Here's how the part is built. I have some questions about the finished solid (model axes, mm). Round coordinates to 2 decimals unless told otherwise and drop trailing zeros. Loops run counter-clockwise (first coordinate to the right, second up) from the corner with the lowest first, then second, coordinate; pieces in that order, holes last. Notation, with made-up numbers: M -19,63 L 3,63 A25 ccw 3,98 Z; hole C -39.5,50 d3. An arc over 180 degrees is marked long. Answer as CSV lines item,"result".
```python
from build123d import *

# Parameters (mm, degrees)
F0_R     = 0.875
F0_R_2   = 0.475
F1_DEPTH = 1.6
F2_DEPTH = 0.25


with BuildPart() as f1:
    # F0 (on Top) → F1 (new body)
    with BuildSketch(Plane.XY):
        Polygon((-5.712371, 40.124945), (-28.712371, 40.124945), (-28.712371, 37.474945), (-28.712371, 34.824945), (-5.712371, 34.824945), (-5.712371, 37.474945), align=None)
        with Locations((-27.27286, 36.149945)):
            Circle(F0_R, mode=Mode.SUBTRACT)
        with Locations((-24.77286, 36.149945)):
            Circle(F0_R, mode=Mode.SUBTRACT)
        with Locations((-22.27286, 36.149945)):
            Circle(F0_R, mode=Mode.SUBTRACT)
        with Locations((-19.77286, 36.149945)):
            Circle(F0_R, mode=Mode.SUBTRACT)
        with Locations((-17.27286, 36.149945)):
            Circle(F0_R, mode=Mode.SUBTRACT)
        with Locations((-14.77286, 36.149945)):
            Circle(F0_R, mode=Mode.SUBTRACT)
        with Locations((-12.27286, 36.149945)):
            Circle(F0_R, mode=Mode.SUBTRACT)
        with Locations((-9.77286, 36.149945)):
            Circle(F0_R, mode=Mode.SUBTRACT)
        with Locations((-7.27286, 36.149945)):
            Circle(F0_R, mode=Mode.SUBTRACT)
        with Locations((-27.264467, 38.799945)):
            Circle(F0_R, mode=Mode.SUBTRACT)
        with Locations((-24.764467, 38.799945)):
            Circle(F0_R, mode=Mode.SUBTRACT)
        with Locations((-22.264467, 38.799945)):
            Circle(F0_R, mode=Mode.SUBTRACT)
        with Locations((-19.764467, 38.799945)):
            Circle(F0_R, mode=Mode.SUBTRACT)
        with Locations((-17.264467, 38.799945)):
            Circle(F0_R, mode=Mode.SUBTRACT)
        with Locations((-14.764467, 38.799945)):
            Circle(F0_R, mode=Mode.SUBTRACT)
        with Locations((-12.264467, 38.799945)):
            Circle(F0_R, mode=Mode.SUBTRACT)
        with Locations((-9.764467, 38.799945)):
            Circle(F0_R, mode=Mode.SUBTRACT)
        with Locations((-7.264467, 38.799945)):
            Circle(F0_R, mode=Mode.SUBTRACT)
        with Locations((-27.264467, 38.799945)):
            Circle(F0_R)
        with Locations((-27.264467, 38.799945)):
            Circle(F0_R_2, mode=Mode.SUBTRACT)
        with Locations((-24.764467, 38.799945)):
            Circle(F0_R)
        with Locations((-24.764467, 38.799945)):
            Circle(F0_R_2, mode=Mode.SUBTRACT)
        with Locations((-22.264467, 38.799945)):
            Circle(F0_R)
        with Locations((-22.264467, 38.799945)):
            Circle(F0_R_2, mode=Mode.SUBTRACT)
        with Locations((-19.764467, 38.799945)):
            Circle(F0_R)
        with Locations((-19.764467, 38.799945)):
            Circle(F0_R_2, mode=Mode.SUBTRACT)
        with Locations((-17.264467, 38.799945)):
            Circle(F0_R)
        with Locations((-17.264467, 38.799945)):
            Circle(F0_R_2, mode=Mode.SUBTRACT)
        with Locations((-14.764467, 38.799945)):
            Circle(F0_R)
        with Locations((-14.764467, 38.799945)):
            Circle(F0_R_2, mode=Mode.SUBTRACT)
        with Locations((-12.264467, 38.799945)):
            Circle(F0_R)
        with Locations((-12.264467, 38.799945)):
            Circle(F0_R_2, mode=Mode.SUBTRACT)
        with Locations((-9.764467, 38.799945)):
            Circle(F0_R)
        with Locations((-9.764467, 38.799945)):
            Circle(F0_R_2, mode=Mode.SUBTRACT)
        with Locations((-7.264467, 38.799945)):
            Circle(F0_R)
        with Locations((-7.264467, 38.799945)):
            Circle(F0_R_2, mode=Mode.SUBTRACT)
        with Locations((-7.27286, 36.149945)):
            Circle(F0_R)
        with Locations((-7.27286, 36.149945)):
            Circle(F0_R_2, mode=Mode.SUBTRACT)
        with Locations((-9.77286, 36.149945)):
            Circle(F0_R)
        with Locations((-9.77286, 36.149945)):
            Circle(F0_R_2, mode=Mode.SUBTRACT)
        with Locations((-12.27286, 36.149945)):
            Circle(F0_R)
        with Locations((-12.27286, 36.149945)):
            Circle(F0_R_2, mode=Mode.SUBTRACT)
        with Locations((-14.77286, 36.149945)):
            Circle(F0_R)
        with Locations((-14.77286, 36.149945)):
            Circle(F0_R_2, mode=Mode.SUBTRACT)
        with Locations((-17.27286, 36.149945)):
            Circle(F0_R)
        with Locations((-17.27286, 36.149945)):
            Circle(F0_R_2, mode=Mode.SUBTRACT)
        with Locations((-19.77286, 36.149945)):
            Circle(F0_R)
        with Locations((-19.77286, 36.149945)):
            Circle(F0_R_2, mode=Mode.SUBTRACT)
        with Locations((-22.27286, 36.149945)):
            Circle(F0_R)
        with Locations((-22.27286, 36.149945)):
            Circle(F0_R_2, mode=Mode.SUBTRACT)
        with Locations((-24.77286, 36.149945)):
            Circle(F0_R)
        with Locations((-24.77286, 36.149945)):
            Circle(F0_R_2, mode=Mode.SUBTRACT)
        with Locations((-27.27286, 36.149945)):
            Circle(F0_R)
        with Locations((-27.27286, 36.149945)):
            Circle(F0_R_2, mode=Mode.SUBTRACT)
    extrude(amount=-F1_DEPTH)

    # F0 (on Top) → F2 (join)
    with BuildSketch(Plane.XY):
        with Locations((-27.264467, 38.799945)):
            Circle(F0_R)
        with Locations((-27.264467, 38.799945)):
            Circle(F0_R_2, mode=Mode.SUBTRACT)
        with Locations((-24.764467, 38.799945)):
            Circle(F0_R)
        with Locations((-24.764467, 38.799945)):
            Circle(F0_R_2, mode=Mode.SUBTRACT)
        with Locations((-22.264467, 38.799945)):
            Circle(F0_R)
        with Locations((-22.264467, 38.799945)):
            Circle(F0_R_2, mode=Mode.SUBTRACT)
        with Locations((-19.764467, 38.799945)):
            Circle(F0_R)
        with Locations((-19.764467, 38.799945)):
            Circle(F0_R_2, mode=Mode.SUBTRACT)
        with Locations((-17.264467, 38.799945)):
            Circle(F0_R)
        with Locations((-17.264467, 38.799945)):
            Circle(F0_R_2, mode=Mode.SUBTRACT)
        with Locations((-14.764467, 38.799945)):
            Circle(F0_R)
        with Locations((-14.764467, 38.799945)):
            Circle(F0_R_2, mode=Mode.SUBTRACT)
        with Locations((-12.264467, 38.799945)):
            Circle(F0_R)
        with Locations((-12.264467, 38.799945)):
            Circle(F0_R_2, mode=Mode.SUBTRACT)
        with Locations((-9.764467, 38.799945)):
            Circle(F0_R)
        with Locations((-9.764467, 38.799945)):
            Circle(F0_R_2, mode=Mode.SUBTRACT)
        with Locations((-27.27286, 36.149945)):
            Circle(F0_R)
        with Locations((-27.27286, 36.149945)):
            Circle(F0_R_2, mode=Mode.SUBTRACT)
        with Locations((-24.77286, 36.149945)):
            Circle(F0_R)
        with Locations((-24.77286, 36.149945)):
            Circle(F0_R_2, mode=Mode.SUBTRACT)
        with Locations((-22.27286, 36.149945)):
            Circle(F0_R)
        with Locations((-22.27286, 36.149945)):
            Circle(F0_R_2, mode=Mode.SUBTRACT)
        with Locations((-19.77286, 36.149945)):
            Circle(F0_R)
        with Locations((-19.77286, 36.149945)):
            Circle(F0_R_2, mode=Mode.SUBTRACT)
        with Locations((-17.27286, 36.149945)):
            Circle(F0_R)
        with Locations((-17.27286, 36.149945)):
            Circle(F0_R_2, mode=Mode.SUBTRACT)
        with Locations((-14.77286, 36.149945)):
            Circle(F0_R)
        with Locations((-14.77286, 36.149945)):
            Circle(F0_R_2, mode=Mode.SUBTRACT)
        with Locations((-12.27286, 36.149945)):
            Circle(F0_R)
        with Locations((-12.27286, 36.149945)):
            Circle(F0_R_2, mode=Mode.SUBTRACT)
        with Locations((-9.77286, 36.149945)):
            Circle(F0_R)
        with Locations((-9.77286, 36.149945)):
            Circle(F0_R_2, mode=Mode.SUBTRACT)
        with Locations((-7.27286, 36.149945)):
            Circle(F0_R)
        with Locations((-7.27286, 36.149945)):
            Circle(F0_R_2, mode=Mode.SUBTRACT)
        with Locations((-7.264467, 38.799945)):
            Circle(F0_R)
        with Locations((-7.264467, 38.799945)):
            Circle(F0_R_2, mode=Mode.SUBTRACT)
    extrude(amount=F2_DEPTH)


solid = f1.part
```
1. I want a section at A-A, the plane x = -19.75. Please give me the cut outline in (y, z), and give its area (3 significant figures).
Evaluation:
outline,"M 34.82,-1.6 L 35.68,-1.6 L 35.68,0.25 L 35.28,0.25 L 35.28,0 L 34.82,0 Z; M 36.62,-1.6 L 38.33,-1.6 L 38.33,0.25 L 37.93,0.25 L 37.93,0 L 37.02,0 L 37.02,0.25 L 36.62,0.25 Z; M 39.27,-1.6 L 40.12,-1.6 L 40.12,0 L 39.67,0 L 39.67,0.25 L 39.27,0.25 Z"
area,"5.84 mm²"
2. I want a section at B-B, the plane z = -0.45. Count the separate pieces of the cut face and the enclosed holes in it, and give its area (3 significant figures).
Evaluation:
separate pieces,"1"
enclosed holes,"18"
area,"109 mm²"
3. If I drill on line 1 (Y direction, x = -22, z = -1.3); line 2 (Y direction, x = -7.5, z = -1); line 3 (Z direction, x = -18.75, y = 35.85), over which ranges is the centre line in solid material (lowest first)? Write a range as [from, to].
Evaluation:
line 1,"y = [34.82, 35.76], [36.54, 38.41], [39.19, 40.12]"
line 2,"y = [34.82, 35.73], [36.57, 38.39], [39.21, 40.12]"
line 3,"z = [-1.6, 0]"
4. We'd pull the mould along Y, two halves only. Please class faces 1 (the cylindrical face through (-27.33, 39.27, -0.69)), 2 (the flat face through (-5.712, 37, -1)): pulls with the +Y half, pulls with the -Y half, needs draft (parallel to the pull), parting line crosses it, or undercut.
Evaluation:
face 1,"undercut"
face 2,"needs draft"
